Check sheet for the drawn part. Datum: minimum x, y, z corner. Units: mm. A direction names the side the tool comes from. Round coordinates to 2 decimals unless told otherwise and drop trailing zeros. Write each loop counter-clockwise with the first axis right and the second up, starting at its lowest first coordinate (ties: lowest second). Pieces come first, ordered by that corner, then holes.
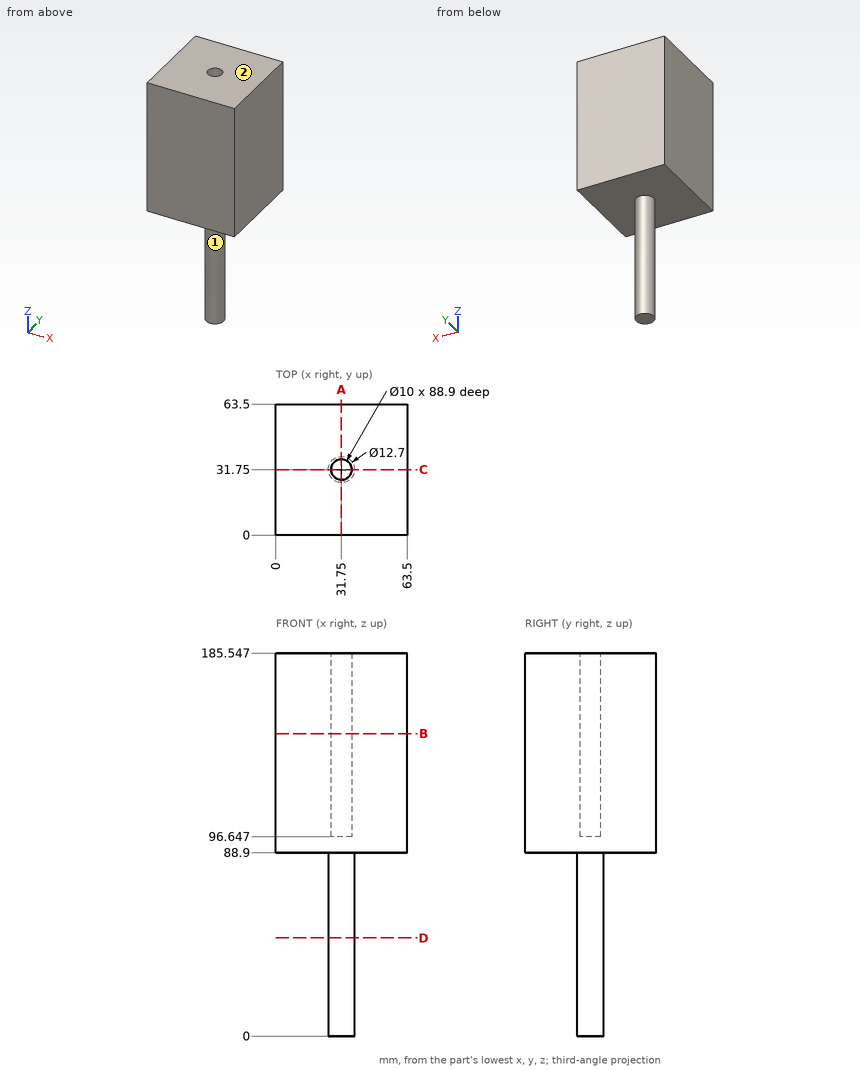
Q1. Depth check by flat-ended pin: P1, Ø4, axis at x = 37, y = 12, coming from the -Z side; P2, Ø5, axis at x = 33.5, y = 32, coming from the +Z side. Enter the tip coordinate at first touch or a pass-through.
Recorded:
P1: stops at z = 88.9
P2: stops at z = 96.65
Q2. Tool access check on the marked faces 1 and 2. Record the directions out of +Z, -Z, +X, -X, +Y, -Y that give a thin tool (end or side, any length) a straight path to the whole face; none if there is none.
Recorded:
face 1: -Z
face 2: +Z, +X, -X, +Y, -Y
Q3. Sectioned sample at D-D (z = 47.5). Enter the section's corners in (x, y), plus the area to 3 significant figures.
Recorded:
outline: circle Ø12.7 at (31.75, 31.75)
area: 127 mm2
Q4. Material ranges on line 1 along Y through (x, z) = (31.75, 145); line 2 along Z through (x, y) = (5, 61), recorded low to high.
Recorded:
line 1: y = 0 to 26.75, 36.75 to 63.5
line 2: z = 88.9 to 185.55
Q5. Sectioned sample at B-B (z = 146.5). Enter the section's corners in (x, y), plus the area to 3 significant figures.
Recorded:
outline: (0, 0) - (63.5, 0) - (63.5, 63.5) - (0, 63.5) - close; hole circle Ø10 at (31.75, 31.75)
area: 3,950 mm2
Q6. Sectioned sample at A-A (x = 31.75). Enter the section's corners in (y, z), plus the area to 3 significant figures.
Recorded:
outline: (0, 88.9) - (25.4, 88.9) - (25.4, 0) - (38.1, 0) - (38.1, 88.9) - (63.5, 88.9) - (63.5, 185.55) - (36.75, 185.55) - (36.75, 96.65) - (26.75, 96.65) - (26.75, 185.55) - (0, 185.55) - close
area: 6,380 mm2
